Design review of the part built by this model. Coordinates are the model's own, in mm. A direction names the side the tool comes from. Round coordinates to 2 decimals unless told otherwise and drop trailing zeros. Order: outer loops, then holes, each group sorted by start corner. A loop starts at its lowest first (then second) coordinate and runs counter-clockwise, first axis right, second up. Notation, with made-up numbers: M 60,-16.75 L 69,-16.75 A16 cw 69,5.25 Z; hole C 28.25,5 d5. An arc over 180 degrees is marked long. Use a Markdown table: item, result. Add a question column.
(1) Take a section at D-D (y = -17). Write out the cut boundary in (x, z), then the cut area to 3 significant figures.
(2) Take a section at C-C (x = 0.5). Write out the cut boundary in (y, z), then the cut area to 3 significant figures.
(3) Take a section at A-A (y = -2.25). Write out the cut boundary in (x, z).
(4) Take a section at B-B (z = -2.75). Write out the cut boundary in (x, y).
(5) Machinability: for faces 5 (the face through (0.27, -3.94, -1.22)), 6 (the face through (2.046, -19.93, -3.25)), 7 (the face through (-3.904, -19.93, -0.19)), 8 (the face through (-2.138, -19.93, 3.245)), 9 (the face through (1.72, -19.93, 3.432)), which of the approach directions +Z, -Z, +X, -X, +Y, -Y give a long, thin tool a straight path to every point of the face, cutting with its end or side? Answer none if there is none.
(6) For pin 1 (5 mm diameter, centred on x = -2, y = -6, fed in from +Z); pin 2 (1.5 mm diameter, centred on y = -14.5, z = 1.5, fed in from -X) (3 decimals); pin 3 (4 mm diameter, centred on x = 4.5, y = -10, fed in from +Z); pin 4 (2 mm diameter, centred on x = 0, z = 0, fed in from +Y), all flat-tipped, find the tip position at first contact; note any pin that passes through.
(7) The part is to be moulded in two halves that separate along Z. For faces 1 (the face through (-4.1, -15, 0.1)), 2 (the face through (-5.854, -7.395, 0.278)), 3 (the face through (0, -8, 0)), 4 (the face through (-1.81, -19.93, -3.44)), say which applies: released by +Z, released by -Z, zero draft, split by the parting line, or undercut.
(8) To check wall thickness, follow probe 1 along Y at (x, z) = (-1, -4.5); probe 2 along Z at (x, y) = (0, -5); probe 3 along X at (y, z) = (-1.5, -1). State the ranges of each line that lie inside material, in increasing order. Write a range as from..to.
```python
from build123d import *

# Parameters (mm, degrees)
F1_DEPTH = 15
F3_DEPTH = 10
F4_R     = 1.25
F5_DEPTH = 8


# Not quite as in the source:
# - ends of sketch curves that miss each other by under 0.0002 mm in the source are joined


with BuildPart() as f1:
    # F0 (on Front) → F1 (new body)
    with BuildSketch(Plane.XZ):
        Polygon((-5.7235665096, 3.5781680242), (-5.9874106989, -3.1166349037), (-0.3214230722, -6.6925111543), (5.608370415, -3.5735600573), (5.8721762755, 3.1212672902), (0.2061886488, 6.6971435408), align=None)
    extrude(amount=F1_DEPTH)

    # F2 (on face) → F3 (join)
    with BuildSketch(Plane.XZ.offset(15)):
        Polygon((-4.0286979474, 2.0048922286), (-3.7759230982, -2.4479388793), (0.2067050986, -4.4554086614), (3.9365390256, -2.0100863602), (3.6837447559, 2.442705723), (-0.2988834409, 4.4501755052), align=None)
    extrude(amount=F3_DEPTH)

    # F4 (on face) → F5 (cut)
    with BuildSketch(Plane(origin=(0, 0, 0), x_dir=(-1, 0, 0), z_dir=(0, 1, 0))):
        Circle(F4_R)
    extrude(amount=-F5_DEPTH, mode=Mode.SUBTRACT)


solid = f1.part
```
Verdict:
| question | item | result |
|---|---|---|
| 1 | outline | M -4.03,2 L -3.78,-2.45 L 0.21,-4.46 L 3.94,-2.01 L 3.68,2.44 L -0.3,4.45 Z |
| 1 | area | 51.7 mm^2 |
| 2 | outline | M -25,-4.26 L -15,-4.26 L -15,-6.26 L 0,-6.26 L 0,-1.15 L -8,-1.15 L -8,1.15 L 0,1.15 L 0,6.51 L -15,6.51 L -15,4.05 L -25,4.05 Z |
| 2 | area | 256 mm^2 |
| 3 | outline | M -5.99,-3.12 L -0.32,-6.69 L 5.61,-3.57 L 5.87,3.12 L 0.21,6.7 L -5.72,3.58 Z; hole C 0,0 d2.5 |
| 4 | outline | M -5.97,-15 L -3.18,-15 L -3.18,-25 L 2.81,-25 L 2.81,-15 L 5.64,-15 L 5.64,0 L -5.97,0 Z |
| 5 | face 5 | +Y |
| 5 | face 6 | -Z, +X, -Y |
| 5 | face 7 | -Z, -X, -Y |
| 5 | face 8 | +Z, -X, -Y |
| 5 | face 9 | +Z, +X, -Y |
| 6 | pin 1 | stops at z = 6.7 |
| 6 | pin 2 | stops at x = -5.835 |
| 6 | pin 3 | stops at z = 5.25 |
| 6 | pin 4 | stops at y = -8 |
| 7 | face 1 | zero draft |
| 7 | face 2 | released by +Z |
| 7 | face 3 | undercut |
| 7 | face 4 | released by -Z |
| 8 | probe 1 | y = -15..0 |
| 8 | probe 2 | z = -6.52..-1.25, 1.25..6.59 |
| 8 | probe 3 | x = -5.9..-0.75, 0.75..5.71 |
